Geometry: final body of the model. Coordinates: model frame, mm. Face numbers are marked on the shaded views. A direction names the side the tool comes from. Coordinates: 2 decimals unless noted, no trailing zeros. Write each loop counter-clockwise with the first axis right and the second up, starting at its lowest first coordinate (ties: lowest second). Pieces come first, ordered by that corner, then holes. Notation, with made-up numbers: M 58.5,-6.75 L 67.5,-6.75 A16 cw 67.5,18.25 Z; hole C -1,-18 d7. An arc over 180 degrees is marked long. Write item = value, one per line. Start each with the question number.
Item 1: Section A-A on x = 5.5. Output: boundary loops of the cut face in (y, z) (3 decimals).
Item 2: Reachability of the marked faces 1, 2, 3, 4 and 5 from +Z, -Z, +X, -X, +Y, -Y: full face, straight path, thin tool, end or side. Return the list, or none.
Item 3: First-contact query: pin 1 Ø4 at (x, z) = (-3.5, 3) entering from +Y; pin 2 Ø3 at (x, z) = (5.5, 2) entering from -Y; pin 3 Ø4 at (x, y) = (1, 9) entering from -Z; pin 4 Ø5 at (y, z) = (0, 0) entering from -X. Flat tips, straight axial feed; report the tip coordinate or a pass-through.
Item 4: Pull-direction query (X, two-part tool) for the marked faces 6, 7 and 8; classes: +X half, -X half, draft (parallel to the pull), parting line (faces both ways), or undercut.
Item 5: Ray query, L1, parallel to Z at x = -4.4, y = 0 (3 decimals); L2, parallel to Z at x = -0.5, y = 0 (3 decimals). Return the intervals inside material, ascending. Write a range as [from, to].
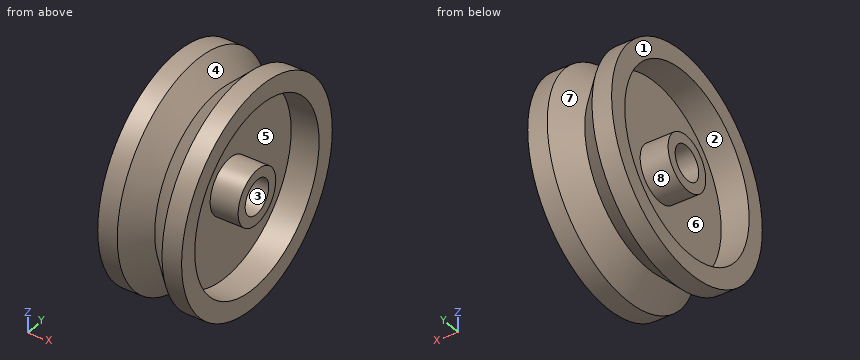
from build123d import *

# Parameters (mm, degrees)
REVOLVE1_ANGLE = 360


with BuildPart() as part:
    # Sketch1 → Revolve1 (revolve, symmetric)
    with BuildSketch(Plane.XY) as revolve1_sk:
        Polygon((7.5, 3.125), (-7.5, 3.125), (-7.5, 5), (-2.5, 5), (-2.5, 16.5), (-7.5, 16.5), (-7.5, 20), (-4, 20), (-0.010995646, 16.000015113), (4, 20), (7.5, 20), (7.5, 16.5), (2.5, 16.5), (2.5, 5), (7.5, 5), align=None)
    revolve(axis=Axis((-7.5, 0, 0), (1, 0, 0)), revolution_arc=REVOLVE1_ANGLE / 2)
    revolve(revolve1_sk.sketch, axis=Axis((-7.5, 0, 0), (-1, 0, 0)), revolution_arc=REVOLVE1_ANGLE / 2)


solid = part.part
Responses:
q1.outline = C 0,0 d40; C 0,0 d10; hole C 0,0 d33; hole C 0,0 d6.25
q2.face_1 = +Z, -Z, -X, +Y, -Y
q2.face_2 = -X
q2.face_3 = +X, -X
q2.face_4 = none
q2.face_5 = +X
q3.pin_1 = 19.97
q3.pin_2 = -19.99
q3.pin_3 = -16.96
q3.pin_4 = through
q4.face_6 = -X half
q4.face_7 = undercut
q4.face_8 = draft
q5.L1 = [-20, -16.5], [-5, -3.125], [3.125, 5], [16.5, 20]
q5.L2 = [-16.49, -3.125], [3.125, 16.49]
